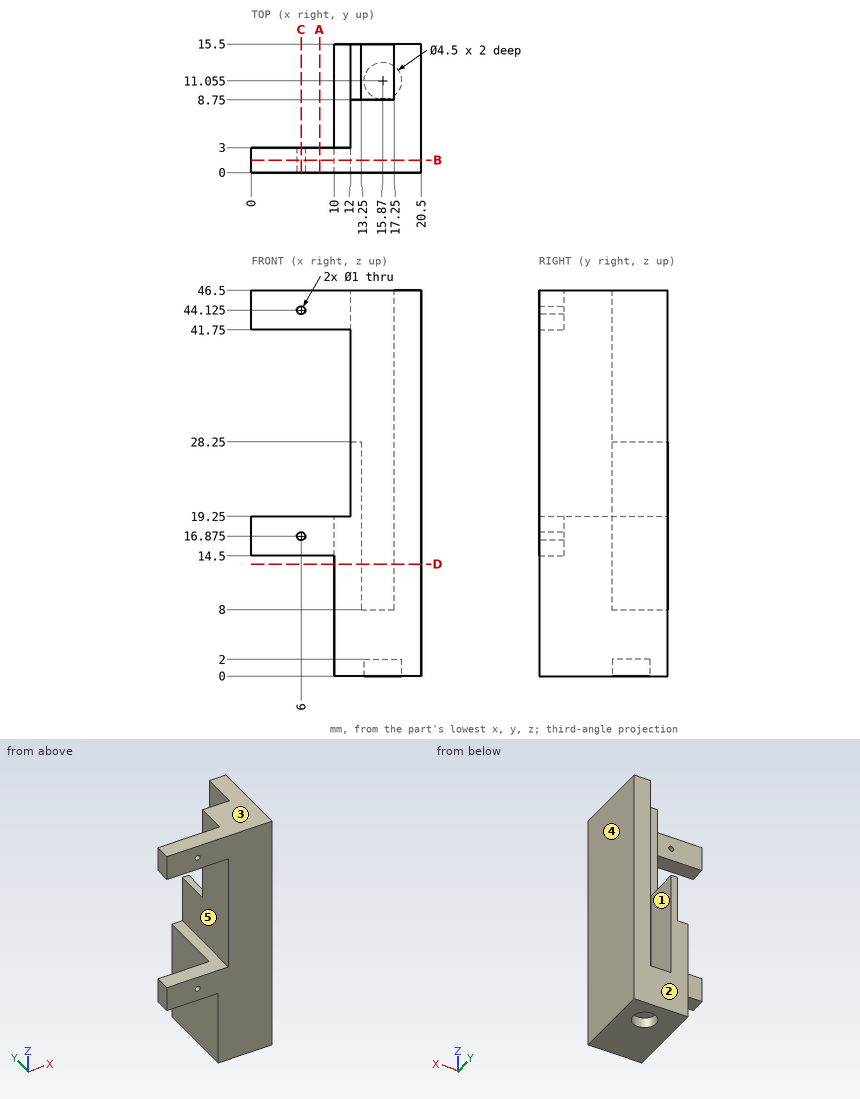
The drawing under review shows one solid part. Ordinate dimensions are in mm from its lowest x, y, z. A direction names the side the tool comes from. Give positions to 0.01 mm unless a question says otherwise; leave off trailing zeros. Order: outer loops, then holes, each group sorted by start corner. A loop starts at its lowest first (then second) coordinate and runs counter-clockwise, first axis right, second up. Notation, with made-up numbers: (29.25, -19.5) - (48.25, -19.5) arc R28 ccw to (48.25, 15.5) - close; hole circle Ø8 at (65.25, 77.25). An arc over 180 degrees is marked (long way). Answer as a JSON object with one key per item and string values. Group by question number.
Item 1: Clearance check with flat-ended pins moving along their axes: pin 1 Ø3 at (x, y) = (10, 14) entering from -Z; pin 2 Ø3.5 at (y, z) = (12.5, 35.5) entering from -X; pin 3 Ø8 at (y, z) = (4, 7) entering from -X; pin 4 Ø2.5 at (x, y) = (3.5, 1.5) entering from -Z. State where each tip first meets the part, or that it passes through.
Item 2: Take a section at D-D on z = 13.5. Give the boundary of the cut face in (x, y), and give its area (3 significant figures).
Item 3: Take a section at B-B on y = 1.5. Give the boundary of the cut face in (x, z) (3 decimals).
Item 4: Machinability: for the marked faces 1 and 2, which of the approach directions +Z, -Z, +X, -X, +Y, -Y give a long, thin tool a straight path to every point of the face, cutting with its end or side? Answer none if there is none.
Item 5: Draft analysis for pull direction Z (two halves, no side actions). For the marked faces 3, 4 and 5, state which applies: pulls with the +Z half, pulls with the -Z half, needs draft (parallel to the pull), parting line crosses it, or undercut.
Item 6: Wall thickness on line 1 along X through (y, z) = (11.75, 11); line 2 along Z through (x, y) = (12.75, 12.75); line 3 along X through (y, z) = (5.75, 21): over which ranges is each line inside the solid? List them lowest first.
Item 7: Take a section at C-C on x = 6. Give the boundary of the cut face in (y, z) (3 decimals), and give its area (3 significant figures).
Item 8: Take a section at A-A on x = 8.25. Give the boundary of the cut face in (y, z).
Reported:
{
 "1": {"pin 1": "z = 0", "pin 2": "x = 17.25", "pin 3": "x = 10", "pin 4": "z = 14.5"},
 "2": {"outline": "(10, 0) - (20.5, 0) - (20.5, 15.5) - (17.25, 15.5) - (17.25, 8.75) - (13.25, 8.75) - (13.25, 15.5) - (10, 15.5) - close", "area": "136 mm^2"},
 "3": {"outline": "(0, 14.5) - (10, 14.5) - (10, 0) - (20.5, 0) - (20.5, 46.5) - (0, 46.5) - (0, 41.75) - (12, 41.75) - (12, 19.25) - (0, 19.25) - close; hole circle Ø1 at (6, 16.875); hole circle Ø1 at (6, 44.125)"},
 "4": {"face 1": "+Z, +Y", "face 2": "+Z, -Z, +X, -X, +Y"},
 "5": {"face 3": "pulls with the +Z half", "face 4": "needs draft", "face 5": "undercut"},
 "6": {"line 1": "10 to 13.25, 17.25 to 20.5", "line 2": "0 to 28.25", "line 3": "12 to 20.5"},
 "7": {"outline": "(0, 14.5) - (3, 14.5) - (3, 16.375) - (0, 16.375) - close; (0, 17.375) - (3, 17.375) - (3, 19.25) - (0, 19.25) - close; (0, 41.75) - (3, 41.75) - (3, 43.625) - (0, 43.625) - close; (0, 44.625) - (3, 44.625) - (3, 46.5) - (0, 46.5) - close", "area": "22.5 mm^2"},
 "8": {"outline": "(0, 14.5) - (3, 14.5) - (3, 19.25) - (0, 19.25) - close; (0, 41.75) - (3, 41.75) - (3, 46.5) - (0, 46.5) - close"}
}
